```python
from build123d import *

# Parameters (mm, degrees)
SKETCH1_R           = 1.5
BOSS_EXTRUDE1_DEPTH = 2
CUT_EXTRUDE2_DEPTH  = 10
FILLET30_R          = 1.5
FILLET31_R          = 5
FILLET32_R          = 2
FILLET33_R          = 3


with BuildPart() as part:
    # Sketch1 → Boss-Extrude1 (new body)
    with BuildSketch(Plane(origin=(0, 0, 0), x_dir=(1, 0, 0), z_dir=(0, 1, 0))):
        Polygon((0, 0), (2, 0), (2, 5), (4, 5), (4, 0), (10, 0), (10, 5), (12, 5), (12, 0), (72.4, 0), (72.4, 5), (74.4, 5), (74.4, 0), (80.4, 0), (80.4, 5), (82.4, 5), (82.4, 0), (84.4, 0), (84.4, 45), (82.4, 45), (82.4, 40), (80.4, 40), (80.4, 45), (74.4, 45), (74.4, 40), (72.4, 40), (72.4, 45), (12, 45), (12, 40), (10, 40), (10, 45), (4, 45), (4, 40), (2, 40), (2, 45), (0, 45), align=None)
        with Locations(Location((7, 42.5, 0), (0, 0, 270))):
            Circle(SKETCH1_R, mode=Mode.SUBTRACT)
        with Locations(Location((77.4, 42.5, 0), (0, 0, 90))):
            Circle(SKETCH1_R, mode=Mode.SUBTRACT)
        with Locations(Location((7, 2.5, 0), (0, 0, 90))):
            Circle(SKETCH1_R, mode=Mode.SUBTRACT)
        with Locations(Location((77.4, 2.5, 0), (0, 0, 270))):
            Circle(SKETCH1_R, mode=Mode.SUBTRACT)
    extrude(amount=BOSS_EXTRUDE1_DEPTH)

    # Sketch3 → Cut-Extrude2 (cut)
    with BuildSketch(Plane(origin=(0, 2, 0), x_dir=(1, 0, 0), z_dir=(0, 1, 0))):
        Polygon((71.845045693, 7.5), (12.554954307, 7.5), (42.2, 19.793561603), align=None)
        Polygon((4.5, 35.427447859), (4.5, 9.572552141), (35.673617122, 22.5), align=None)
        Polygon((12.554954307, 37.5), (42.2, 25.206438397), (71.845045693, 37.5), align=None)
        Polygon((79.9, 35.427447859), (79.9, 9.572552141), (48.726382878, 22.5), align=None)
    extrude(amount=-CUT_EXTRUDE2_DEPTH, mode=Mode.SUBTRACT)

    # Fillet30
    fillet30_edges = [part.edges().sort_by_distance(p)[0] for p in [
        (12.554954307, 1, -7.5),
        (71.845045693, 1, -7.5),
        (71.845045693, 1, -37.5),
        (12.554954307, 1, -37.5),
    ]]
    fillet(fillet30_edges, radius=FILLET30_R)

    # Fillet31
    fillet31_edges = [part.edges().sort_by_distance(p)[0] for p in [
        (42.2, 1, -19.793561603),
        (42.2, 1, -25.206438397),
    ]]
    fillet(fillet31_edges, radius=FILLET31_R)

    # Fillet32
    fillet32_edges = [part.edges().sort_by_distance(p)[0] for p in [
        (35.673617122, 1, -22.5),
        (48.726382878, 1, -22.5),
    ]]
    fillet(fillet32_edges, radius=FILLET32_R)

    # Fillet33
    fillet33_edges = [part.edges().sort_by_distance(p)[0] for p in [
        (4.5, 1, -9.572552141),
        (4.5, 1, -35.427447859),
        (79.9, 1, -35.427447859),
        (79.9, 1, -9.572552141),
    ]]
    fillet(fillet33_edges, radius=FILLET33_R)


solid = part.part
```
The listing builds one solid part. Answer for the finished solid, in the listing's coordinates (mm). A direction names the side the tool comes from. Round coordinates to 2 decimals unless told otherwise and drop trailing zeros. Order: outer loops, then holes, each group sorted by start corner. A loop starts at its lowest first (then second) coordinate and runs counter-clockwise, first axis right, second up. Notation, with made-up numbers: (-25, -38) -> (-8, -38) arc R28 cw to (-8, -12) -> close; hole circle Ø7 at (-5.75, -32). An arc over 180 degrees is marked (long way). Answer as CSV lines item,"result".
Q1. For a pull along Z with two mould halves and no side action, classify faces 1 (the flat face through (42, 2, -23)), 2 (the flat face through (3, 1, -40)), 3 (the flat face through (29.75, 1.01, -14.63)), 4 (the cylindrical face through (78.532, 0.986, -33.453)) as +Z half, -Z half, draft (parallel to the pull), parting line (faces both ways), or undercut.
Computed values:
face 1,"draft"
face 2,"-Z half"
face 3,"undercut"
face 4,"undercut"
Q2. A cutting plane is placed at C-C on x = 37.5. Determine the outline of the cut face in (y, z).
Computed values:
outline,"(0, -45) -> (2, -45) -> (2, -37.5) -> (0, -37.5) -> close; (0, -27.16) -> (2, -27.16) -> (2, -17.84) -> (0, -17.84) -> close; (0, -7.5) -> (2, -7.5) -> (2, 0) -> (0, 0) -> close"
Q3. A cutting plane is placed at B-B on x = 77.4. Determine the outline of the cut face in (y, z).
Computed values:
outline,"(0, -45) -> (2, -45) -> (2, -44) -> (0, -44) -> close; (0, -41) -> (2, -41) -> (2, -33.89) -> (0, -33.89) -> close; (0, -11.11) -> (2, -11.11) -> (2, -4) -> (0, -4) -> close; (0, -1) -> (2, -1) -> (2, 0) -> (0, 0) -> close"
Q4. Consider line 1 (X direction, y = 1.5, z = -40.5); line 2 (X direction, y = 1.75, z = -33.5); line 3 (Z direction, x = 21, y = 0.1). Determine where each line is inside the solid, lowest interval first. Write a range as from..to.
Computed values:
line 1,"x = 0..2, 4..10, 12..72.4, 74.4..80.4, 82.4..84.4"
line 2,"x = 0..5.94, 9.15..22.2, 62.2..75.25, 78.46..84.4"
line 3,"z = -45..-37.5, -34..-28.59, -16.41..-11, -7.5..0"
Q5. Given pin 1 (0.6 mm diameter, centred on x = 52, y = 1, fed in from +Z); pin 2 (1 mm diameter, centred on x = 73.5, y = 1.5, fed in from +Z), each flat-ended and moving along its own axis, determine where each tip first touches the part or whether it passes through.
Computed values:
pin 1,"stops at z = 0"
pin 2,"stops at z = -5"
Q6. Which of the six approach directions +Z, -Z, +X, -X, +Y, -Y give full straight-line access (tool end or side, diameter ignored) to faces 5 (the flat face through (74.4, 1, -3)), 6 (the flat face through (4, 1, -43)), 7 (the flat face through (7, 1, -45)), 8 (the cylindrical face through (51.948, 0.986, -22.533))?
Computed values:
face 5,"+Z, +Y, -Y"
face 6,"-Z, +Y, -Y"
face 7,"-Z, +X, -X, +Y, -Y"
face 8,"+Y, -Y"
Q7. A cutting plane is placed at D-D on z = -27.5. Determine the outline of the cut face in (x, y).
Computed values:
outline,"(0, 0) -> (4.5, 0) -> (4.5, 2) -> (0, 2) -> close; (23.62, 0) -> (36.67, 0) -> (36.67, 2) -> (23.62, 2) -> close; (47.73, 0) -> (60.78, 0) -> (60.78, 2) -> (47.73, 2) -> close; (79.9, 0) -> (84.4, 0) -> (84.4, 2) -> (79.9, 2) -> close"
Q8. A cutting plane is placed at A-A on z = -2.5. Determine the outline of the cut face in (x, y).
Computed values:
outline,"(0, 0) -> (2, 0) -> (2, 2) -> (0, 2) -> close; (4, 0) -> (5.5, 0) -> (5.5, 2) -> (4, 2) -> close; (8.5, 0) -> (10, 0) -> (10, 2) -> (8.5, 2) -> close; (12, 0) -> (72.4, 0) -> (72.4, 2) -> (12, 2) -> close; (74.4, 0) -> (75.9, 0) -> (75.9, 2) -> (74.4, 2) -> close; (78.9, 0) -> (80.4, 0) -> (80.4, 2) -> (78.9, 2) -> close; (82.4, 0) -> (84.4, 0) -> (84.4, 2) -> (82.4, 2) -> close"
